```python
from build123d import *

# Parameters (mm, degrees)
F1_R     = 42
F2_DEPTH = 3
F3_DEPTH = 3
F6_DEPTH = 30


# Not quite as in the source:
# - a fillet or chamfer that OpenCascade refuses, or shapes differently, is made with other operations: its cross-section is extruded or revolved along the edge and cut away or added


with BuildPart() as f2:
    # F1 (on Top) → F2 (new body)
    with BuildSketch(Plane.XY):
        with Locations((9.5, 0)):
            Circle(F1_R)
    extrude(amount=F2_DEPTH)

    # F0 (on Top) → F3 (cut)
    with BuildSketch(Plane.XY):
        with BuildLine():
            Line((6, 0), (13, 0))
            ThreePointArc((13, 0), (9.5, 3.5), (6, 0))
        make_face()
        with BuildLine():
            ThreePointArc((6, 0), (9.5, -3.5), (13, 0))
            Line((13, 0), (6, 0))
        make_face()
    extrude(amount=F3_DEPTH, mode=Mode.SUBTRACT)

    # F4: fillet of radius 4 on 1 edges, made by hand

    # F4_s1 → F4_t2 (revolve, cut)
    with BuildSketch(Plane.XZ):
        with BuildLine():
            ThreePointArc((51.5, 0), (50.0765063966, 2.1622776602), (47.6270166538, 3))
            Line((47.6270166538, 3), (51.5, 3))
            Line((51.5, 3), (51.5, 0))
        make_face()
    revolve(axis=Axis((9.5, 0, 3), (0, 0, 1)), mode=Mode.SUBTRACT)

    # F5 (on face) → F6 (cut)
    with BuildSketch(Plane.XY):
        with BuildLine():
            Line((-13.7163735325, 19), (32.7163735325, 19))
            ThreePointArc((32.7163735325, 19), (9.5, 30), (-13.7163735325, 19))
        make_face()
        with BuildLine():
            Line((32.7163735325, -19), (-13.7163735325, -19))
            ThreePointArc((-13.7163735325, -19), (9.5, -30), (32.7163735325, -19))
        make_face()
    extrude(amount=F6_DEPTH, mode=Mode.SUBTRACT)


solid = f2.part
```
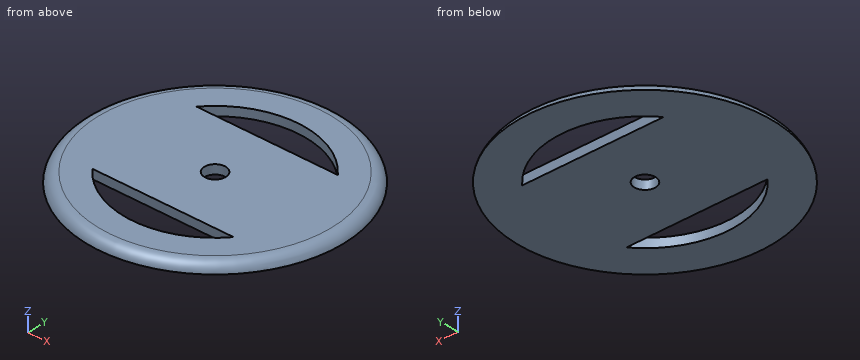
Build history of the part. All positions in model axes, mm. Give positions to 0.01 mm unless a question says otherwise; leave off trailing zeros. Order: outer loops, then holes, each group sorted by start corner. A loop starts at its lowest first (then second) coordinate and runs counter-clockwise, first axis right, second up. Notation, with made-up numbers: M 66,44.5 L 73,44.5 A23 cw 73,59.5 Z; hole C 67.25,82 d11. An arc over 180 degrees is marked long. Write item = value, one per line. Start each with the question number.
(1) Slice it at C-C on z = 0.65. Write the cut outline in (x, y).
(2) Pin check, flat tips, straight feed: pin 1 Ø1.5 at (y, z) = (-25, 1) entering from -X; pin 2 Ø1 at (x, z) = (40, 1) entering from -Y; pin 3 Ø9 at (x, y) = (9.5, 0) entering from +Z. Stop position of each tip, or through.
(3) Probe L1, parallel to Y at x = 1, z = 0.1; L2, parallel to Y at x = 4, z = 1.6; L3, parallel to Y at x = 10, z = 1.1. List the from-to ranges inside material, lowest first. Write a range as [from, to].
(4) Slice it at A-A on y = 0. Write the cut outline in (x, z), plus the area to 3 significant figures.
(5) Slice it at B-B on x = 9.5. Write the cut outline in (y, z), plus the area to 3 significant figures.
(6) Slice it at D-D on x = -5. State how many separate pieces and enclosed holes the cut face has, plus the area to 3 significant figures.
Responses:
q1.outline = C 9.5,0 d83.54; hole M -13.72,-19 A30 ccw 32.72,-19 Z; hole M -13.72,19 L 32.72,19 A30 ccw Z; hole C 9.5,0 d7
q2.pin_1 = -24.46
q2.pin_2 = -28.93
q2.pin_3 = 3
q3.L1 = [-41.1, -28.77], [-19, 19], [28.77, 41.1]
q3.L2 = [-40.8, -29.49], [-19, 19], [29.49, 40.8]
q3.L3 = [-41.53, -30], [-19, -3.46], [3.46, 19], [30, 41.53]
q4.outline = M -32.5,0 L 6,0 L 6,3 L -28.63,3 A4 ccw Z; M 13,0 L 51.5,0 A4 ccw 47.63,3 L 13,3 Z
q4.area = 225 mm2
q5.outline = M -42,0 L -30,0 L -30,3 L -38.13,3 A4 ccw Z; M -19,0 L -3.5,0 L -3.5,3 L -19,3 Z; M 3.5,0 L 19,0 L 19,3 L 3.5,3 Z; M 30,0 L 42,0 A4 ccw 38.13,3 L 30,3 Z
q5.area = 159 mm2
q6.separate_pieces = 3
q6.enclosed_holes = 0
q6.area = 186 mm2
